```python
from build123d import *

# Parameters (mm, degrees)
MODEL_R             = 0.5
MODEL_R_2           = 1.25
BOSS_EXTRUDE1_DEPTH = 1.6


with BuildPart() as part:
    # Model → Boss-Extrude1 (new body)
    with BuildSketch(Plane.XY):
        with BuildLine():
            Line((0, 15.24), (0, 2.54))
            ThreePointArc((0, 2.54), (0.743948776, 0.743948776), (2.54, 0))
            Line((2.54, 0), (22.86, 0))
            ThreePointArc((22.86, 0), (24.656051224, 0.743948776), (25.4, 2.54))
            Line((25.4, 2.54), (25.4, 15.24))
            ThreePointArc((25.4, 15.24), (24.656051224, 17.036051224), (22.86, 17.78))
            Line((22.86, 17.78), (2.54, 17.78))
            ThreePointArc((2.54, 17.78), (0.743948776, 17.036051224), (0, 15.24))
        make_face()
        with Locations((6.35, 2.54)):
            Circle(MODEL_R, mode=Mode.SUBTRACT)
        with Locations((8.89, 2.54)):
            Circle(MODEL_R, mode=Mode.SUBTRACT)
        with Locations((11.43, 2.54)):
            Circle(MODEL_R, mode=Mode.SUBTRACT)
        with Locations((13.97, 2.54)):
            Circle(MODEL_R, mode=Mode.SUBTRACT)
        with Locations((16.51, 2.54)):
            Circle(MODEL_R, mode=Mode.SUBTRACT)
        with Locations((19.05, 2.54)):
            Circle(MODEL_R, mode=Mode.SUBTRACT)
        with Locations((16.51, 15.24)):
            Circle(MODEL_R, mode=Mode.SUBTRACT)
        with Locations((19.05, 15.24)):
            Circle(MODEL_R, mode=Mode.SUBTRACT)
        with Locations((6.35, 15.24)):
            Circle(MODEL_R, mode=Mode.SUBTRACT)
        with Locations((8.89, 15.24)):
            Circle(MODEL_R, mode=Mode.SUBTRACT)
        with Locations((2.54, 15.24)):
            Circle(MODEL_R_2, mode=Mode.SUBTRACT)
        with Locations((22.86, 15.24)):
            Circle(MODEL_R_2, mode=Mode.SUBTRACT)
        with Locations((2.54, 2.54)):
            Circle(MODEL_R_2, mode=Mode.SUBTRACT)
        with Locations((22.86, 2.54)):
            Circle(MODEL_R_2, mode=Mode.SUBTRACT)
        with Locations((10.9, 13.97)):
            Circle(MODEL_R, mode=Mode.SUBTRACT)
        with Locations((14.4, 13.97)):
            Circle(MODEL_R, mode=Mode.SUBTRACT)
    extrude(amount=-BOSS_EXTRUDE1_DEPTH)


solid = part.part
```
The model under review builds one solid part; all positions refer to its coordinate system, in mm. Give positions to 0.01 mm unless a question says otherwise; leave off trailing zeros. Write each loop counter-clockwise with the first axis right and the second up, starting at its lowest first coordinate (ties: lowest second). Pieces come first, ordered by that corner, then holes. Notation, with made-up numbers: M 83.5,-21.5 L 95.5,-21.5 A19 cw 95.5,-6.5 Z; hole C 6,-12 d11. An arc over 180 degrees is marked long. Answer in a Markdown table with one row per item.
Item 1: Add section C-C on y = 3.5. Give the boundary of the cut face in (x, z).
Check sheet entries:
| item | result |
|---|---|
| outline | M 0,-1.6 L 1.74,-1.6 L 1.74,0 L 0,0 Z; M 3.34,-1.6 L 22.06,-1.6 L 22.06,0 L 3.34,0 Z; M 23.66,-1.6 L 25.4,-1.6 L 25.4,0 L 23.66,0 Z |
Item 2: Draft analysis for pull direction X (two halves, no side actions). For faces 1 (the face through (10.835, 14.466, -0.789)), 2 (the face through (24.636, 0.724, -0.789)), 3 (the face through (13, 17.78, -1)), 4 (the face through (16.402, 2.052, -0.789)), state which applies: +X half, -X half, draft (parallel to the pull), parting line (faces both ways), or undercut.
Check sheet entries:
| item | result |
|---|---|
| face 1 | undercut |
| face 2 | +X half |
| face 3 | draft |
| face 4 | undercut |
Item 3: Add section A-A on x = 19.05. Give the boundary of the cut face in (y, z), plus the area to 3 significant figures.
Check sheet entries:
| item | result |
|---|---|
| outline | M 0,-1.6 L 2.04,-1.6 L 2.04,0 L 0,0 Z; M 3.04,-1.6 L 14.74,-1.6 L 14.74,0 L 3.04,0 Z; M 15.74,-1.6 L 17.78,-1.6 L 17.78,0 L 15.74,0 Z |
| area | 25.2 mm2 |
Item 4: For line 1 along Y through (x, z) = (16.51, -1.2); line 2 along Y through (x, z) = (14.4, -0.65); line 3 along X through (y, z) = (3.25, -1.25), list the stretches that pass through material, from the lowest coordinate up.
Check sheet entries:
| item | result |
|---|---|
| line 1 | 0 to 2.04, 3.04 to 14.74, 15.74 to 17.78 |
| line 2 | 0 to 2.28, 2.8 to 13.47, 14.47 to 17.78 |
| line 3 | 0 to 1.51, 3.57 to 21.83, 23.89 to 25.4 |
Item 5: Add section B-B on z = -0.5. State how many separate pieces and enclosed holes the cut face has, plus the area to 3 significant figures.
Check sheet entries:
| item | result |
|---|---|
| separate pieces | 1 |
| enclosed holes | 16 |
| area | 417 mm2 |
